Could you check a few things on this model? Use its own coordinates, in mm. A direction names the side the tool comes from. Give positions to 0.01 mm unless a question says otherwise; leave off trailing zeros. Loops run counter-clockwise (first coordinate to the right, second up) from the corner with the lowest first, then second, coordinate; pieces in that order, holes last. Notation, with made-up numbers: (52.5, 52) - (84.5, 52) arc R29 ccw to (84.5, 81) - close; hole circle Ø11 at (-35, 51). An arc over 180 degrees is marked (long way). Write each question's results on one line, items separated by ' | '. Start each with the question number.
1) If I drill on probe 1 along X at (y, z) = (-0.25, -3); probe 2 along Z at (x, y) = (-3, -6.75), over which ranges is the centre line in solid material (lowest first)? Write a range as [from, to].
2) I'm going to push flat-ended pins straight in: pin 1 (8 mm diameter, centred on x = -2, z = -11.5, fed in from +Y); pin 2 (6 mm diameter, centred on x = 8.5, z = 23, fed in from +Y); pin 3 (4 mm diameter, centred on y = 1.5, z = 22, fed in from +X). Where does each tip first touch, or does it pass through?
3) I want a section at C-C, the plane z = 7. Write out the boundary of the cut face in (x, y), and give its area (3 significant figures).
4) I want a section at B-B, the plane y = 0. Write out the boundary of the cut face in (x, z).
5) I want a section at D-D, the plane y = -8.25. Write out the boundary of the cut face in (x, z), and give its area (3 significant figures).
6) I want a section at A-A, the plane x = 0. Write out the boundary of the cut face in (y, z).
7) On a 3-axis mill with a long thin cutter (end or side, diameter ignored), from which of +Z, -Z, +X, -X, +Y, -Y can I reach the whole of each face in a straight line? I mean faces 1 (the face through (-9.714, 0, -10)), 2 (the face through (0, -4.828, -10)), 3 (the face through (0, 8, 39)), 4 (the face through (0, 4.828, -10)), 5 (the face through (-2.17, -9.76, 24.16)). Say none if no direction works.
from build123d import *

# Parameters (mm, degrees)
SKETCH1_R           = 10
BOSS_EXTRUDE1_DEPTH = 49
SKETCH2_R           = 12
BOSS_EXTRUDE2_DEPTH = 5
CUT_EXTRUDE1_DEPTH  = 10
SKETCH4_W           = 19.428573608
SKETCH4_H           = 9.65531402
BOSS_EXTRUDE3_DEPTH = 10


with BuildPart() as part:
    # Sketch1 → Boss-Extrude1 (new body)
    with BuildSketch(Plane.XY):
        Circle(SKETCH1_R)
    extrude(amount=BOSS_EXTRUDE1_DEPTH)

    # Sketch2 → Boss-Extrude2 (add)
    with BuildSketch(Plane(origin=(0, 0, 0), x_dir=(-1, 0, 0), z_dir=(0, 0, -1))):
        Circle(SKETCH2_R)
    extrude(amount=BOSS_EXTRUDE2_DEPTH)

    # Sketch3 → Cut-Extrude1 (cut)
    with BuildSketch(Plane.XY.offset(49)):
        with BuildLine():
            Line((0, 6), (8, 6))
            ThreePointArc((8, 6), (0, 10), (-8, 6))
            Line((-8, 6), (0, 6))
        make_face()
    extrude(amount=-CUT_EXTRUDE1_DEPTH, mode=Mode.SUBTRACT)

    # Sketch4 → Boss-Extrude3 (add)
    with BuildSketch(Plane(origin=(0, 0, -5), x_dir=(-1, 0, 0), z_dir=(0, 0, -1))):
        Rectangle(SKETCH4_W, SKETCH4_H)
    extrude(amount=BOSS_EXTRUDE3_DEPTH)


solid = part.part
Answers:
1) probe 1: x = [-12, 12] | probe 2: z = [-5, 49]
2) pin 1: stops at y = 4.83 | pin 2: stops at y = 8.35 | pin 3: stops at x = 10
3) outline: circle Ø20 at (0, 0) | area: 314 mm2
4) outline: (-12, -5) - (-9.71, -5) - (-9.71, -15) - (9.71, -15) - (9.71, -5) - (12, -5) - (12, 0) - (10, 0) - (10, 49) - (-10, 49) - (-10, 0) - (-12, 0) - close
5) outline: (-8.71, -5) - (8.71, -5) - (8.71, 0) - (5.65, 0) - (5.65, 49) - (-5.65, 49) - (-5.65, 0) - (-8.71, 0) - close | area: 641 mm2
6) outline: (-12, -5) - (-4.83, -5) - (-4.83, -15) - (4.83, -15) - (4.83, -5) - (12, -5) - (12, 0) - (10, 0) - (10, 39) - (6, 39) - (6, 49) - (-10, 49) - (-10, 0) - (-12, 0) - close
7) face 1: -Z, -X, +Y, -Y | face 2: -Z, +X, -X, -Y | face 3: +Z, +X, -X, +Y | face 4: -Z, +X, -X, +Y | face 5: +Z
